```python
from build123d import *

# Parameters (mm, degrees)
SKETCH_1_W          = 197
SKETCH_1_H          = 229
EXTRUDE_1_DEPTH     = 2.7
SKETCH_2_R          = 1.1
CUT_EXTRUDE_1_DEPTH = 2.85
SKETCH_3_R          = 1.35
CUT_EXTRUDE_2_DEPTH = 9
SKETCH_5_R          = 1.75
CUT_EXTRUDE_3_DEPTH = 10
SKETCH_6_W          = 20
SKETCH_6_H          = 80
SKETCH_6_H_2        = 150
CUT_EXTRUDE_4_DEPTH = 10
FILLET_1_R          = 5


with BuildPart() as part:
    # 草图1 → 凸台-拉伸1 (new body)
    with BuildSketch(Plane.XY):
        with Locations((98.5, 114.5)):
            Rectangle(SKETCH_1_W, SKETCH_1_H)
    extrude(amount=EXTRUDE_1_DEPTH)

    # 草图2 → 切除-拉伸1 (cut)
    with BuildSketch(Plane.XY.offset(2.7)):
        with Locations((4, 4)):
            Circle(SKETCH_2_R)
        with Locations((193, 4)):
            Circle(SKETCH_2_R)
    extrude(amount=-CUT_EXTRUDE_1_DEPTH, mode=Mode.SUBTRACT)

    # 草图3 → 切除-拉伸2 (cut)
    with BuildSketch(Plane(origin=(0, 0, 0), x_dir=(-1, 0, 0), z_dir=(0, 0, -1))):
        with Locations((-133.1, 12.9)):
            Circle(SKETCH_3_R)
        with Locations((-133.1, 82.1)):
            Circle(SKETCH_3_R)
        with Locations((-63.9, 82.1)):
            Circle(SKETCH_3_R)
        with Locations((-63.9, 12.9)):
            Circle(SKETCH_3_R)
    extrude(amount=-CUT_EXTRUDE_2_DEPTH, mode=Mode.SUBTRACT)

    # 草图5 → 切除-拉伸3 (cut)
    with BuildSketch(Plane(origin=(0, 0, 0), x_dir=(-1, 0, 0), z_dir=(0, 0, -1))):
        with Locations((-132.5, 214)):
            Circle(SKETCH_5_R)
        with Locations((-64.501425834, 213.559646274)):
            Circle(SKETCH_5_R)
        with Locations((-132.5, 123.4)):
            Circle(SKETCH_5_R)
        with Locations((-64.5, 122.959646285)):
            Circle(SKETCH_5_R)
    extrude(amount=-CUT_EXTRUDE_3_DEPTH, mode=Mode.SUBTRACT)

    # 草图6 → 切除-拉伸4 (cut)
    with BuildSketch(Plane(origin=(0, 0, 0), x_dir=(-1, 0, 0), z_dir=(0, 0, -1))):
        with Locations((-168.5, 114.5)):
            Rectangle(SKETCH_6_W, SKETCH_6_H)
        with Locations((-28.5, 114.5)):
            Rectangle(SKETCH_6_W, SKETCH_6_H)
        with Locations((-98.5, 114.5)):
            Rectangle(SKETCH_6_W, SKETCH_6_H_2)
    extrude(amount=-CUT_EXTRUDE_4_DEPTH, mode=Mode.SUBTRACT)

    # 圆角1
    fillet_1_edges = [part.edges().sort_by_distance(p)[0] for p in [
        (178.5, 74.5, 1.35),
        (178.5, 154.5, 1.35),
        (158.5, 154.5, 1.35),
        (158.5, 74.5, 1.35),
        (38.5, 74.5, 1.35),
        (38.5, 154.5, 1.35),
        (18.5, 154.5, 1.35),
        (18.5, 74.5, 1.35),
        (108.5, 39.5, 1.35),
        (108.5, 189.5, 1.35),
        (88.5, 189.5, 1.35),
        (88.5, 39.5, 1.35),
    ]]
    fillet(fillet_1_edges, radius=FILLET_1_R)


solid = part.part
```
For this review, take the finished solid that the model builds, in its own axes (mm). A direction names the side the tool comes from. Round coordinates to 2 decimals unless told otherwise and drop trailing zeros. Write each loop counter-clockwise with the first axis right and the second up, starting at its lowest first coordinate (ties: lowest second). Pieces come first, ordered by that corner, then holes. Notation, with made-up numbers: (9.25, 75.25) - (29.25, 75.25) arc R26 ccw to (29.25, 110.25) - close; hole circle Ø2 at (74.25, 1). An arc over 180 degrees is marked (long way). Put each result on its own line as item: value.
Q1. Wall thickness on probe 1 along X at (y, z) = (82.1, 1.45); probe 2 along X at (y, z) = (97, 2); probe 3 along Y at (x, z) = (133.1, 2.05): over which ranges is each line inside the solid? List them lowest first.
Solved:
probe 1: x = 0 to 18.5, 38.5 to 62.55, 65.25 to 88.5, 108.5 to 131.75, 134.45 to 158.5, 178.5 to 197
probe 2: x = 0 to 18.5, 38.5 to 88.5, 108.5 to 158.5, 178.5 to 197
probe 3: y = 0 to 11.55, 14.25 to 80.75, 83.45 to 121.76, 125.04 to 212.36, 215.64 to 229
Q2. Mouldability with a two-part tool opening along Y and no side actions: class faces 1 (the face through (37.07, 153, 1.37)), 2 (the face through (160, 153.07, 1.37)), 3 (the face through (119, 116, 2.7)) as released by +Y, released by -Y, zero draft, split by the parting line, or undercut.
Solved:
face 1: undercut
face 2: undercut
face 3: zero draft
Q3. We need section A-A (y = 69). Give the boundary of the cut face in (x, z).
Solved:
outline: (0, 0) - (88.5, 0) - (88.5, 2.7) - (0, 2.7) - close; (108.5, 0) - (197, 0) - (197, 2.7) - (108.5, 2.7) - close
Q4. Insertion check: pin 1 Ø1.8 at (x, y) = (4, 4) entering from -Z. The pin has a flat end and moves straight along its axis. Give the tip position at first contact, or say it passes through.
Solved:
pin 1: passes through
Q5. We need section C-C (y = 135). Give the boundary of the cut face in (x, z).
Solved:
outline: (0, 0) - (18.5, 0) - (18.5, 2.7) - (0, 2.7) - close; (38.5, 0) - (88.5, 0) - (88.5, 2.7) - (38.5, 2.7) - close; (108.5, 0) - (158.5, 0) - (158.5, 2.7) - (108.5, 2.7) - close; (178.5, 0) - (197, 0) - (197, 2.7) - (178.5, 2.7) - close
Q6. Machinability: for faces 4 (the face through (177.07, 76, 1.37)), 5 (the face through (119, 116, 0)), which of the approach directions +Z, -Z, +X, -X, +Y, -Y give a long, thin tool a straight path to every point of the face, cutting with its end or side? Answer none if there is none.
Solved:
face 4: +Z, -Z
face 5: -Z, +X, -X, +Y, -Y
Q7. We need section D-D (z = 2). Count the separate pieces of the cut face and the enclosed holes in it, and give its area (3 significant figures).
Solved:
separate pieces: 1
enclosed holes: 13
area: 38,900 mm2
Q8. We need section B-B (x = 168). Give the boundary of the cut face in (y, z), and give its area (3 significant figures).
Solved:
outline: (0, 0) - (74.5, 0) - (74.5, 2.7) - (0, 2.7) - close; (154.5, 0) - (229, 0) - (229, 2.7) - (154.5, 2.7) - close
area: 402 mm2
